Could you check a few things on this model? Use its own coordinates, in mm. A direction names the side the tool comes from. Give positions to 0.01 mm unless a question says otherwise; leave off trailing zeros. Loops run counter-clockwise (first coordinate to the right, second up) from the corner with the lowest first, then second, coordinate; pieces in that order, holes last. Notation, with made-up numbers: M 27,46.25 L 78,46.25 A19 cw 78,72.25 Z; hole C -2.75,-19 d8. An arc over 180 degrees is marked long. Return JSON: item names as keys, results as strings. Group by question number.
1. If we section it at B-B (y = 0): Write out the boundary of the cut face in (x, z).
2. For pin 1 (1.6 mm diameter, centred on x = 0.5, y = 4.5, fed in from -Z); pin 2 (0.8 mm diameter, centred on x = 4.5, z = -0.5, fed in from -Y); pin 3 (3 mm diameter, centred on x = -3.5, y = 0, fed in from +Z), each with a flat end and sliding along its axis, tell me the tip position at first contact or that it passes through.
3. If we mould it in two halves opening along X, with no side actions, what happens to faces 1 (the cylindrical face through (-5.25, -0.08, -0.11)), 2 (the cylindrical face through (8.43, -7.4, 1.97)), 3 (the flat face through (0, -8, 2))? For each: +X half, -X half, draft (parallel to the pull), parting line (faces both ways), or undercut.
4. If we section it at C-C (z = 3.7): Write out the boundary of the cut face in (x, y), plus the area to 3 significant figures.
5. For faces 4 (the cylindrical face through (-5.9, 1.8, 3)), 5 (the flat face through (-8.5, 0, -0.5)), 6 (the cylindrical face through (3.77, -0.08, 0.55)), 7 (the flat face through (0.1, -2.8, -0.5)), 8 (the flat face through (0, 5, 0)), which set-ups out of +Z, -Z, +X, -X, +Y, -Y let a thin tool reach every point of the face, with its end or its side?
6. Please list where these lines run through material, in increasing order: line 1 (Y direction, x = -3.5, z = 3.5); line 2 (X direction, y = 0, z = 3); line 3 (X direction, y = 1.5, z = 3.15).
7. If we section it at D-D (x = 6.5): Write out the boundary of the cut face in (y, z), plus the area to 3 significant figures.
8. If we section it at A-A (x = -3.5): Write out the boundary of the cut face in (y, z).
Autodesk Fusion 360 part; units mm, degrees
sketch "Sketch1" plane through (0, 0, 0) normal (0, 0, 1) x (1, 0, 0)
  line L0 (9, 8) -> (-9, 8)
  line L1 (-9, 8) -> (-9, -8)
  line L2 (-9, -8) -> (9, -8)
  line L3 (9, -8) -> (9, 8)
  circle A0 centre (-3.5, 0) radius 1.75
  circle A1 centre (-3.5, 0) radius 3
  line L4 (9, -2.8) -> (-9, -2.8)
  line L5 (-9, -2.8) -> (-9, 2.8)
  line L6 (-9, 2.8) -> (9, 2.8)
  line L7 (9, 2.8) -> (9, -2.8)
  line L8 (9, -2.8) -> (-9, 2.8) construction
  line L9 (-9, -2.8) -> (9, 2.8) construction
  dimension "d1" = 18
  dimension "d2" = 16
  dimension "d5" = 3.5
  dimension "d6" = 6
  dimension "d9" = 5.6
  dimension "d12" = 3.5
  dimension "d23" = 8
extrude "Extrude1" add sketch "Sketch1" along normal blind 2
extrude "Extrude2" add sketch "Sketch1" along normal blind 4 contours L0 L1 L3 A1 L6 | L3 A1 L4 L6 L7 | L1 A1 L4 L5 L6 | L1 L2 L3 A1 L4
extrude "Extrude3" add sketch "Sketch1" against normal blind 1 contours L3 A1 L4 L6 L7 | L1 A1 L4 L5 L6 | A1 L4 L6
sketch "Sketch2" plane through (9, 0, 0) normal (1, 0, 0) x (0, 1, 0)
  line L0 (-8, 0) -> (-2.8, 0)
  line L1 (-2.8, 0) -> (-2.8, -1)
  line L2 (-2.8, -1) -> (2.8, -1)
  line L3 (2.8, -1) -> (2.8, 0)
  line L4 (2.8, 0) -> (8, 0)
  line L5 (8, 0) -> (8, 4)
  line L6 (8, 4) -> (-8, 4)
  line L7 (-8, 4) -> (-8, 0)
  circle A0 centre (0, 5) radius 2.25
  circle A1 centre (0, 5) radius 4.45
  line L8 (-8, 0) -> (8, 0)
  line L9 (0, 4) -> (0, 5) construction
  dimension "d13" = 4.5
  dimension "d14" = 2.2
  dimension "d18" = 5
extrude "Extrude4" cut sketch "Sketch2" against normal blind 3.5 from surface at -3.5 contours L6 A0 A1 picked at (-0.2762, 1.3019)
chamfer "Chamfer1" distance 1.2 angle 45 1 edges at (-5.1316, 0.6328, 2)
fillet "Fillet1" radius 2 4 edges at (-9, -8, 2) (9, -8, 2) (9, 8, 2) (-9, 8, 2)
chamfer "Chamfer2" distance 1 angle 45 2 edges at (-9, 0, -1) (9, 0, -1)
equation "d23 = d2 / 2"
Answer:
{
 "1": {"outline": "M -9,0 L -8,-1 L -5.25,-1 L -5.25,0.8 L -6.45,2 L -6.5,2 L -6.5,4 L -9,4 Z; M -1.75,-1 L 8,-1 L 9,0 L 9,4 L -0.5,4 L -0.5,2 L -0.55,2 L -1.75,0.8 Z; hole M 2,0.55 L 5.5,0.55 L 5.5,2.75 L 2,2.75 Z"},
 "2": {"pin 1": "stops at z = 0", "pin 2": "stops at y = -2.8", "pin 3": "passes through"},
 "3": {"face 1": "undercut", "face 2": "+X half", "face 3": "draft"},
 "4": {"outline": "M -9,-6 A2 ccw -7,-8 L 7,-8 A2 ccw 9,-6 L 9,6 A2 ccw 7,8 L -7,8 A2 ccw -9,6 Z; hole C -3.5,0 d6; hole M 2,-4.26 L 5.5,-4.26 L 5.5,-1.84 L 2,-1.84 Z; hole M 2,1.84 L 5.5,1.84 L 5.5,4.26 L 2,4.26 Z", "area": "239 mm²"},
 "5": {"face 4": "+Z", "face 5": "-Z, -X, +Y, -Y", "face 6": "none", "face 7": "-Z, +X, -X, -Y", "face 8": "-Z, +X, -X, +Y"},
 "6": {"line 1": "y = -8 to -3, 3 to 8", "line 2": "x = -9 to -6.5, -0.5 to 9", "line 3": "x = -9 to -6.1, -0.9 to 2, 5.5 to 9"},
 "7": {"outline": "M -8,0 L -2.8,0 L -2.8,-1 L 2.8,-1 L 2.8,0 L 8,0 L 8,4 L -8,4 Z", "area": "69.6 mm²"},
 "8": {"outline": "M -8,0 L -2.8,0 L -2.8,-1 L -1.75,-1 L -1.75,0.8 L -2.95,2 L -3,2 L -3,4 L -8,4 Z; M 1.75,-1 L 2.8,-1 L 2.8,0 L 8,0 L 8,4 L 3,4 L 3,2 L 2.95,2 L 1.75,0.8 Z"}
}
